Part model, mm, in its own coordinate system. A direction names the side the tool comes from. Give positions to 0.01 mm unless a question says otherwise; leave off trailing zeros. Order: outer loops, then holes, each group sorted by start corner. A loop starts at its lowest first (then second) coordinate and runs counter-clockwise, first axis right, second up. Notation, with made-up numbers: M -9,-36.75 L -5,-36.75 A10 ccw -5,-24.75 Z; hole C -20.5,50.25 d3. An arc over 180 degrees is marked long. Return JSON: item names as keys, results as strings.
Autodesk Inventor part; units mm, degrees
ref_plane "YZ Plane" through (0, 0, 0) normal (1, 0, 0) x (0, 1, 0)
ref_plane "XZ Plane" through (0, 0, 0) normal (0, 1, 0) x (-1, 0, 0)
ref_plane "XY Plane" through (0, 0, 0) normal (0, 0, 1) x (1, 0, 0)
sketch "Náčrt1" plane through (0, 0, 0) normal (0, 0, 1) x (1, 0, 0)
  line L0 (0, 0) -> (14, 0)
  line L1 (14, 0) -> (14, 25)
  line L2 (14, 25) -> (0, 25)
  line L3 (0, 25) -> (0, 0)
  circle A0 centre (7, 7) radius 2.5
  point P0 (7, 0)
  dimension "d0" = 14
  dimension "d1" = 25
  dimension "d2" = 5
  dimension "d3" = 7
  dimension "d4" = 7
extrude "Vysunutí1" add sketch "Náčrt1" against normal blind 4
sketch "Náčrt2" plane through (0, 0, 0) normal (0, 0, 1) x (1, 0, 0)
  line L0 (0, 0) -> (0, 25)
  line L1 (14, 25) -> (14, 0)
  line L2 (0, 25) -> (14, 25)
  line L3 (14, 25) -> (14, 21)
  line L4 (14, 21) -> (0, 21)
  line L5 (0, 21) -> (0, 25)
  point P0 (0, 21)
  dimension "d7" = 4
extrude "Vysunutí2" add sketch "Náčrt2" along normal blind 14
fillet "Zaoblení1" radius 3 1 edges at (7, 21, 0)
fillet "Zaoblení2" radius 3 2 edges at (0, 0, -2) (14, 0, -2)
chamfer "Zkosení1" distance 1 angle 45 2 edges at (0, 23, 14) (14, 23, 14)
properties part number "Packa" material "Zlatá"
Q1. Band-saw the part on B-B (x = 7). Give the cut face in (y, z).
Established:
{"outline": "M 0,-4 L 4.5,-4 L 4.5,0 L 0,0 Z; M 9.5,-4 L 25,-4 L 25,14 L 21,14 L 21,3 A3 cw 18,0 L 9.5,0 Z"}
Q2. Probe line 1 along Y through (x, z) = (7, -1.8); line 2 along Y through (x, z) = (5.5, 6.5); line 3 along Z through (x, y) = (5.5, 11.5). List the from-to ranges inside material, lowest first.
Established:
{"line 1": "y = 0 to 4.5, 9.5 to 25", "line 2": "y = 21 to 25", "line 3": "z = -4 to 0"}
Q3. Band-saw the part on A-A (y = 5). Give the cut face in (x, z), then the cut area to 3 significant figures.
Established:
{"outline": "M 0,-4 L 5.5,-4 L 5.5,0 L 0,0 Z; M 8.5,-4 L 14,-4 L 14,0 L 8.5,0 Z", "area": "44.0 mm²"}
Q4. 3-axis set-ups, long thin cutter, end or side, ignore diameter. For faces 1 (the flat face through (7, 21, 8)), 2 (the flat face through (13.5, 23, 13.5)): which of +Z, -Z, +X, -X, +Y, -Y reach the whole face in a straight line?
Established:
{"face 1": "+Z, +X, -X, -Y", "face 2": "+Z, +X, +Y, -Y"}
Q5. Pin check, flat tips, straight feed: pin 1 (2 mm diameter, centred on y = 4, z = 2.5, fed in from -X); pin 2 (2 mm diameter, centred on x = 2.5, z = 6, fed in from -Y); pin 3 (4 mm diameter, centred on x = 6, y = 9, fed in from +Z). Stop position of each tip, or through.
Established:
{"pin 1": "passes through", "pin 2": "stops at y = 21", "pin 3": "stops at z = 0"}
Q6. Band-saw the part on C-C (z = -2). Give the cut face in (x, y), then the cut area to 3 significant figures.
Established:
{"outline": "M 0,3 A3 ccw 3,0 L 11,0 A3 ccw 14,3 L 14,25 L 0,25 Z; hole C 7,7 d5", "area": "327 mm²"}
Q7. Band-saw the part on D-D (x = 10.5). Give the cut face in (y, z), then the cut area to 3 significant figures.
Established:
{"outline": "M 0,-4 L 25,-4 L 25,14 L 21,14 L 21,3 A3 cw 18,0 L 0,0 Z", "area": "158 mm²"}
